from build123d import *

# Parameters (mm, degrees)
BOSS_EXTRUDE1_DEPTH = 25
SKETCH2_R           = 0.95
CUT_EXTRUDE1_DEPTH  = 25
CHAMFER1_SIZE       = 5
FILLET1_R           = 1
CHAMFER2_SIZE       = 0.3


with BuildPart() as part:
    # Sketch1 → Boss-Extrude1 (new body)
    with BuildSketch(Plane(origin=(0, 0, 0), x_dir=(1, 0, 0), z_dir=(0, 1, 0))):
        Polygon((0, 0), (-18.35, 0), (-18.35, -3.475), (-28.35, -3.475), (-28.35, -8.475), (-15.65, -8.475), (-15.65, -5), (0, -5), align=None)
    extrude(amount=BOSS_EXTRUDE1_DEPTH)

    # Sketch2 → Cut-Extrude1 (cut)
    with BuildSketch(Plane.XY.offset(5)):
        with Locations((-7.65, 4.5)):
            Circle(SKETCH2_R)
        with Locations((-7.65, 19.5)):
            Circle(SKETCH2_R)
    extrude(amount=-CUT_EXTRUDE1_DEPTH, mode=Mode.SUBTRACT)

    # Chamfer1
    chamfer1_edges = [part.edges().sort_by_distance(p)[0] for p in [
        (-28.35, 25, 5.975),
        (-28.35, 0, 5.975),
    ]]
    chamfer(chamfer1_edges, length=CHAMFER1_SIZE)

    # Fillet1
    fillet1_edges = [part.edges().sort_by_distance(p)[0] for p in [
        (-18.35, 0, 1.7375),
        (0, 0, 2.5),
        (-18.35, 25, 1.7375),
        (-15.65, 25, 6.7375),
        (-28.35, 20, 5.975),
        (-28.35, 5, 5.975),
        (-23.35, 0, 5.975),
        (-23.35, 25, 5.975),
        (0, 25, 2.5),
        (-15.65, 0, 6.7375),
    ]]
    fillet(fillet1_edges, radius=FILLET1_R)

    # Chamfer2
    chamfer2_edges = [part.edges().sort_by_distance(p)[0] for p in [
        (-20.642893219, 0, 3.475),
        (-20.642893219, 25, 3.475),
        (-8.6, 4.5, 0),
        (-8.6, 4.5, 5),
        (-8.6, 19.5, 0),
        (-8.6, 19.5, 5),
        (-8.325, 25, 5),
        (-19.792893219, 25, 8.475),
        (-9.175, 25, 0),
        (-15.65, 12.5, 8.475),
        (-28.35, 12.5, 8.475),
        (-25.85, 2.5, 8.475),
        (-19.792893219, 0, 8.475),
        (-25.85, 22.5, 8.475),
        (-28.273879533, 5.03153013, 8.475),
        (-23.31846987, 0.076120467, 8.475),
        (-15.942893219, 0.292893219, 8.475),
        (-28.273879533, 19.96846987, 8.475),
        (-23.31846987, 24.923879533, 8.475),
        (-15.942893219, 24.707106781, 8.475),
        (-25.85, 22.5, 3.475),
        (-25.85, 2.5, 3.475),
        (-28.35, 12.5, 3.475),
        (-28.273879533, 5.03153013, 3.475),
        (-23.31846987, 0.076120467, 3.475),
        (-28.273879533, 19.96846987, 3.475),
        (-23.31846987, 24.923879533, 3.475),
        (-9.175, 0, 0),
        (-18.35, 12.5, 0),
        (0, 12.5, 0),
        (-0.292893219, 0.292893219, 0),
        (-18.057106781, 0.292893219, 0),
        (-18.057106781, 24.707106781, 0),
        (-0.292893219, 24.707106781, 0),
        (0, 12.5, 5),
        (-0.292893219, 0.292893219, 5),
        (-0.292893219, 24.707106781, 5),
        (-8.325, 0, 5),
    ]]
    chamfer(chamfer2_edges, length=CHAMFER2_SIZE)


solid = part.part
Model file for the job. Use its own axes, mm. A direction names the side the tool comes from. Round coordinates to 2 decimals unless told otherwise and drop trailing zeros. Loops run counter-clockwise (first coordinate to the right, second up) from the corner with the lowest first, then second, coordinate; pieces in that order, holes last.
1. Tool access for faces 1 (the flat face through (-15.65, 12, 7)), 2 (the flat face through (-12, 0, 3)), 3 (the flat face through (-18.35, 12, 2)), 4 (the flat face through (-25.71, 2.58, 8.33)), 5 (the cylindrical face through (-18.065, 24.699, 2.062)): list every direction of +Z, -Z, +X, -X, +Y, -Y with a clear straight run to the whole face (end or side of a thin tool).
Check values:
face 1: +Z, +X, +Y, -Y
face 2: +Z, -Z, +X, -X, -Y
face 3: -Z, -X, +Y, -Y
face 4: +Z, -X, -Y
face 5: -Z, -X, +Y
2. Mould opens along X. For faces 6 (the cylindrical face through (-7.856, 18.573, 2.531)), 7 (the cylindrical face through (-15.951, 0.285, 6.413)), 8 (the conical face through (-17.932, 0.43, 0.115)) say: +X half, -X half, draft (parallel to the pull), parting line (faces both ways), or undercut.
Check values:
face 6: undercut
face 7: +X half
face 8: -X half
3. Wall check: probe 1 along Y at (x, z) = (-7.65, 3.85); probe 2 along Z at (x, y) = (-15.5, 1); probe 3 along X at (y, z) = (5.5, 2.5). Give the ranges that are in metal, low to high.
Check values:
probe 1: y = 0 to 3.55, 5.45 to 18.55, 20.45 to 25
probe 2: z = 0 to 5
probe 3: x = -18.35 to 0
4. Drop flat-ended pins along their axis: P1, Ø4.5, axis at x = -8.5, y = 8, coming from the +Z side; P2, Ø4, axis at y = 13.5, z = 2, coming from the -X side; P3, Ø2.5, axis at y = 14.5, z = 6.5, coming from the +X side; P4, Ø1, axis at y = 13.5, z = 2.5, coming from the -X side. Give the stop position or say it passes through.
Check values:
P1: stops at z = 5
P2: stops at x = -28.35
P3: stops at x = -15.65
P4: stops at x = -18.35
5. Band-saw the part on A-A, the plane x = -7.65. List the corners of the cut face in (y, z), and give its area (3 significant figures).
Check values:
outline: (0, 0.3) - (0.3, 0) - (3.25, 0) - (3.55, 0.3) - (3.55, 4.7) - (3.25, 5) - (0.3, 5) - (0, 4.7) - close; (5.45, 0.3) - (5.75, 0) - (18.25, 0) - (18.55, 0.3) - (18.55, 4.7) - (18.25, 5) - (5.75, 5) - (5.45, 4.7) - close; (20.45, 0.3) - (20.75, 0) - (24.7, 0) - (25, 0.3) - (25, 4.7) - (24.7, 5) - (20.75, 5) - (20.45, 4.7) - close
area: 105 mm2
6. Band-saw the part on B-B, the plane z = 7.5. List the corners of the cut face in (x, y).
Check values:
outline: (-28.35, 5.41) arc R1 ccw to (-28.06, 4.71) - (-23.64, 0.29) arc R1 ccw to (-22.94, 0) - (-16.65, 0) arc R1 ccw to (-15.65, 1) - (-15.65, 24) arc R1 ccw to (-16.65, 25) - (-22.94, 25) arc R1 ccw to (-23.64, 24.71) - (-28.06, 20.29) arc R1 ccw to (-28.35, 19.59) - close
7. Band-saw the part on C-C, the plane y = 8. List the corners of the cut face in (x, z) (3 decimals).
Check values:
outline: (-28.35, 3.775) - (-28.05, 3.475) - (-18.35, 3.475) - (-18.35, 0.3) - (-18.05, 0) - (-0.3, 0) - (0, 0.3) - (0, 4.7) - (-0.3, 5) - (-15.65, 5) - (-15.65, 8.175) - (-15.95, 8.475) - (-28.05, 8.475) - (-28.35, 8.175) - close
8. Band-saw the part on D-D, the plane x = -14.75. List the corners of the cut face in (y, z).
Check values:
outline: (0, 0.3) - (0.3, 0) - (24.7, 0) - (25, 0.3) - (25, 4.7) - (24.7, 5) - (0.3, 5) - (0, 4.7) - close
